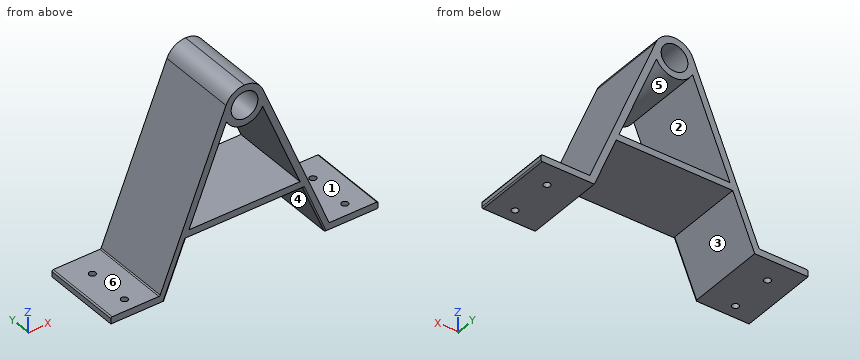
```python
from build123d import *

# Parameters (mm, degrees)
F0_R     = 10
F1_DEPTH = 60
F2_R     = 2.5
F3_DEPTH = 5.001
F4_R     = 1


with BuildPart() as f1:
    # F0 (on Front) → F1 (new body)
    with BuildSketch(Plane.XZ):
        with BuildLine():
            ThreePointArc((86.1209118397, 120.6895440801), (85.0074372508, 114.5277053764), (86.5065387851, 108.4481678561))
            ThreePointArc((86.5065387851, 108.4481678561), (100, 100), (113.4934612149, 108.4481678561))
            ThreePointArc((113.4934612149, 108.4481678561), (114.9925627492, 114.5277053764), (113.8790881603, 120.6895440801))
            ThreePointArc((113.8790881603, 120.6895440801), (108.356340072, 127.4567885348), (100, 130))
            ThreePointArc((100, 130), (91.643659928, 127.4567885348), (86.1209118397, 120.6895440801))
        make_face()
        with Locations((100, 115)):
            Circle(F0_R, mode=Mode.SUBTRACT)
        with BuildLine():
            Line((58.4471400894, 40), (86.5065387851, 108.4481678561))
            ThreePointArc((86.5065387851, 108.4481678561), (85.0074372508, 114.5277053764), (86.1209118397, 120.6895440801))
            Line((86.1209118397, 120.6895440801), (36.6458690181, 0))
            Line((36.6458690181, 0), (0, 0))
            Line((0, 0), (0, -5))
            Line((0, -5), (40, -5))
            Line((40, -5), (56.3974578573, 35))
            Line((56.3974578573, 35), (143.6025421427, 35))
            Line((143.6025421427, 35), (160, -5))
            Line((160, -5), (200, -5))
            Line((200, -5), (200, 0))
            Line((200, 0), (163.3541309819, 0))
            Line((163.3541309819, 0), (113.8790881603, 120.6895440801))
            ThreePointArc((113.8790881603, 120.6895440801), (114.9925627492, 114.5277053764), (113.4934612149, 108.4481678561))
            Line((113.4934612149, 108.4481678561), (141.5528599106, 40))
            Line((141.5528599106, 40), (58.4471400894, 40))
        make_face()
    extrude(amount=-F1_DEPTH)

    # F2 (on face) → F3 (cut, through all)
    with BuildSketch(Plane.XY):
        with Locations((182.5, 10)):
            Circle(F2_R)
        with Locations((182.5, 42.5)):
            Circle(F2_R)
        with Locations((17.5, 10)):
            Circle(F2_R)
        with Locations((17.5, 42.5)):
            Circle(F2_R)
    extrude(amount=-F3_DEPTH, mode=Mode.SUBTRACT)

    # F4
    f4_edges = [f1.edges().sort_by_distance(p)[0] for p in [
        (200, 30, 0),
        (200, 30, -5),
        (0, 30, 0),
        (151.801271, 0, 15),
        (48.198729, 0, 15),
        (36.645869, 30, 0),
    ]]
    fillet(f4_edges, radius=F4_R)


solid = f1.part
```
The listing builds one solid part. Answer for the finished solid, in the listing's coordinates (mm). Face numbers are marked on the shaded views. A direction names the side the tool comes from. Coordinates: 2 decimals unless noted, no trailing zeros. Write each loop counter-clockwise with the first axis right and the second up, starting at its lowest first coordinate (ties: lowest second). Pieces come first, ordered by that corner, then holes. Notation, with made-up numbers: M 75,47 L 94,47 A15 cw 94,70 Z; hole C 75.25,11 d6. An arc over 180 degrees is marked long. Use a Markdown table: item, result. Add a question column.
1. Section D-D (z = 48.5) is taken. Give the vertices of the cut face in (x, y).
2. Straight lines are drawn through the part: line 1 along Y through (x, z) = (17, -2); line 2 along Z through (x, y) = (101, 41.5); line 3 along X through (y, z) = (42, -3). For each, find the intervals that lie inside material, in ascending order. Write a range as [from, to].
3. For a pull along Z with two mould halves and no side action, classify the marked faces 4, 5 and 6 as +Z half, -Z half, draft (parallel to the pull), parting line (faces both ways), or undercut.
4. Given P1, Ø10, axis at x = 99, y = 33.5, coming from the -Z side; P2, Ø4, axis at x = 50, y = 15.5, coming from the -Z side; P3, Ø10, axis at x = 49.5, y = 14.5, coming from the +Z side; P4, Ø3, axis at x = 17.5, y = 42.5, coming from the +Z side, each flat-ended and moving along its own axis, determine where each tip first touches the part or whether it passes through.
5. Section A-A (y = 10) is taken. Count the separate pieces of the cut face and the enclosed holes in it, plus the area to 3 significant figures.
6. Which of the six approach directions +Z, -Z, +X, -X, +Y, -Y give full straight-line access (tool end or side, diameter ignored) to the marked faces 1, 2 and 3?
7. Section B-B (x = 17.5) is taken. Give the vertices of the cut face in (y, z).
8. Section C-C (y = 30) is taken. Give the vertices of the cut face in (x, z).
Data:
| question | item | result |
|---|---|---|
| 1 | outline | M 56.53,0 L 61.93,0 L 61.93,60 L 56.53,60 Z; M 138.07,0 L 143.47,0 L 143.47,60 L 138.07,60 Z |
| 2 | line 1 | y = [0, 7.55], [12.45, 40.05], [44.95, 60] |
| 2 | line 2 | z = [35, 40], [100.03, 105.05], [124.95, 129.97] |
| 2 | line 3 | x = [0, 15.05], [19.95, 40.82], [159.18, 180.05], [184.95, 200] |
| 3 | face 4 | -Z half |
| 3 | face 5 | undercut |
| 3 | face 6 | +Z half |
| 4 | P1 | stops at z = 35 |
| 4 | P2 | stops at z = 14.52 |
| 4 | P3 | stops at z = 43.55 |
| 4 | P4 | passes through |
| 5 | separate pieces | 3 |
| 5 | enclosed holes | 2 |
| 5 | area | 2,390 mm2 |
| 6 | face 1 | +Z, +X, +Y, -Y |
| 6 | face 2 | +Y, -Y |
| 6 | face 3 | -Z, +Y, -Y |
| 7 | outline | M 0,-5 L 7.5,-5 L 7.5,0 L 0,0 Z; M 12.5,-5 L 40,-5 L 40,0 L 12.5,0 Z; M 45,-5 L 60,-5 L 60,0 L 45,0 Z |
| 8 | outline | M 0,-5 L 40,-5 L 56.4,35 L 143.6,35 L 160,-5 L 199,-5 A1 ccw 200,-4 L 200,-1 A1 ccw 199,0 L 163.35,0 L 113.88,120.69 A15 ccw 86.12,120.69 L 36.9,0.62 A1 cw 35.98,0 L 1,0 A1 ccw 0,-1 Z; hole M 58.45,40 L 141.55,40 L 113.49,108.45 A15 cw 86.51,108.45 Z; hole C 100,115 d20 |
